```python
from build123d import *

# Parameters (mm, degrees)
SKETCH1_R           = 10
SKETCH1_R_2         = 2
BOSS_EXTRUDE1_DEPTH = 2
SKETCH2_R           = 4.5
SKETCH2_R_2         = 3.5
BOSS_EXTRUDE2_DEPTH = 2


with BuildPart() as part:
    # Sketch1 → Boss-Extrude1 (new body)
    with BuildSketch(Plane.XY):
        Circle(SKETCH1_R)
        with Locations((7, 0)):
            Circle(SKETCH1_R_2, mode=Mode.SUBTRACT)
        with Locations((0, 7)):
            Circle(SKETCH1_R_2, mode=Mode.SUBTRACT)
        with Locations((-7, 0)):
            Circle(SKETCH1_R_2, mode=Mode.SUBTRACT)
        with Locations((0, -7)):
            Circle(SKETCH1_R_2, mode=Mode.SUBTRACT)
    extrude(amount=BOSS_EXTRUDE1_DEPTH)

    # Sketch2 → Boss-Extrude2 (add)
    with BuildSketch(Plane(origin=(0, 0, 0), x_dir=(-1, 0, 0), z_dir=(0, 0, -1))):
        Circle(SKETCH2_R)
        Circle(SKETCH2_R_2, mode=Mode.SUBTRACT)
    extrude(amount=BOSS_EXTRUDE2_DEPTH)


solid = part.part
```
The model under review builds one solid part; all positions refer to its coordinate system, in mm. A direction names the side the tool comes from. Give positions to 0.01 mm unless a question says otherwise; leave off trailing zeros. Write each loop counter-clockwise with the first axis right and the second up, starting at its lowest first coordinate (ties: lowest second). Pieces come first, ordered by that corner, then holes.
(1) Consider section C-C, the plane y = 7. Give the boundary of the cut face in (x, z), and give its area (3 significant figures).
(2) The part is to be moulded in two halves that separate along Y. For faces 3 (the flat face through (0, 0, 0)), 4 (the cylindrical face through (0.59, 4.46, -0.99)), 5 (the flat face through (4.3, -2.1, 0)), say which applies: released by +Y, released by -Y, zero draft, split by the parting line, or undercut.
(3) For P1, Ø6.5, axis at x = 0, y = 0, coming from the -Z side; P2, Ø3.5, axis at x = 0, y = -7, coming from the -Z side; P3, Ø1, axis at y = 1.5, z = -1, coming from the +X side, all flat-tipped, find the tip position at first contact; note any pin that passes through.
(4) To check wall thickness, follow L1, parallel to Y at x = 0, z = 0.65; L2, parallel to Y at x = 0, z = -1.5; L3, parallel to Y at x = -1.75, z = 0.65. State the ranges of each line that lie inside material, in increasing order.
(5) Consider section D-D, the plane x = 5.25. Give the boundary of the cut face in (y, z), and give its area (3 significant figures).
(6) Consider section B-B, the plane y = 0. Give the boundary of the cut face in (x, z).
(7) Consider section A-A, the plane z = 0.25. Give the boundary of the cut face in (x, y).
(8) Tool access review of faces 1 (the flat face through (0, -4, -2)), 2 (the cylindrical face through (-3.233, -1.341, -0.986)): name each direction out of +Z, -Z, +X, -X, +Y, -Y from which nothing blocks a thin tool from reaching the whole face with its end or side.
Returned:
1. outline: (-7.14, 0) - (-2, 0) - (-2, 2) - (-7.14, 2) - close; (2, 0) - (7.14, 0) - (7.14, 2) - (2, 2) - close
1. area: 20.6 mm2
2. face 3: undercut
2. face 4: split by the parting line
2. face 5: zero draft
3. P1: stops at z = 0
3. P2: passes through
3. P3: stops at x = 4.39
4. L1: y = -10 to -9, -5 to 5, 9 to 10
4. L2: y = -4.5 to -3.5, 3.5 to 4.5
4. L3: y = -9.85 to -7.97, -6.03 to 6.03, 7.97 to 9.85
5. outline: (-8.51, 0) - (-0.97, 0) - (-0.97, 2) - (-8.51, 2) - close; (0.97, 0) - (8.51, 0) - (8.51, 2) - (0.97, 2) - close
5. area: 30.2 mm2
6. outline: (-10, 0) - (-9, 0) - (-9, 2) - (-10, 2) - close; (-5, 0) - (-4.5, 0) - (-4.5, -2) - (-3.5, -2) - (-3.5, 0) - (3.5, 0) - (3.5, -2) - (4.5, -2) - (4.5, 0) - (5, 0) - (5, 2) - (-5, 2) - close; (9, 0) - (10, 0) - (10, 2) - (9, 2) - close
7. outline: circle Ø20 at (0, 0); hole circle Ø4 at (-7, 0); hole circle Ø4 at (0, -7); hole circle Ø4 at (0, 7); hole circle Ø4 at (7, 0)
8. face 1: -Z, +X, -X, +Y, -Y
8. face 2: -Z
